```python
from build123d import *

# Parameters (mm, degrees)
F0_W     = 50
F0_H     = 25
F1_DEPTH = 10
F2_R     = 4
F3_W     = 5
F3_H     = 15
F4_DEPTH = 25
F5_R     = 1
F6_R     = 3.6231488333
F6_R_2   = 2.5645914907
F7_DEPTH = 1.5


with BuildPart() as f1:
    # F0 (on Top) → F1 (new body)
    with BuildSketch(Plane.XY):
        Rectangle(F0_W, F0_H)
    extrude(amount=F1_DEPTH)

    # F2
    f2_edges = [f1.edges().sort_by_distance(p)[0] for p in [
        (-25, -12.5, 5),
        (25, -12.5, 5),
        (25, 12.5, 5),
        (-25, 12.5, 5),
    ]]
    fillet(f2_edges, radius=F2_R)

    # F3 (on face) → F4 (cut)
    with BuildSketch(Plane.XY.offset(10)):
        with Locations((-18.5, 0)):
            Rectangle(F3_W, F3_H)
    extrude(amount=-F4_DEPTH, mode=Mode.SUBTRACT)

    # F5
    f5_edges = [f1.edges().sort_by_distance(p)[0] for p in [
        (-21, 7.5, 5),
        (-21, -7.5, 5),
        (-16, 7.5, 5),
        (-16, -7.5, 5),
    ]]
    fillet(f5_edges, radius=F5_R)

    # F6 (on face) → F7 (join)
    with BuildSketch(Plane.XY.offset(10)):
        with BuildLine():
            ThreePointArc((0, -8.4754349664), (4.4343331639, -0.0092051923), (0, 8.4570245817))
            ThreePointArc((0, 8.4570245817), (-4.7324505421, -0.0092051923), (0, -8.4754349664))
        make_face()
        with BuildLine():
            ThreePointArc((0, -7.3103578761), (-3.8122546037, 0.107302476), (0, 7.524962828))
            ThreePointArc((0, 7.524962828), (3.6492929607, 0.107302476), (0, -7.3103578761))
        make_face(mode=Mode.SUBTRACT)
        Circle(F6_R)
        Circle(F6_R_2, mode=Mode.SUBTRACT)
        with BuildLine():
            Line((-7.5879783359, -7.5879783359), (-3.4245205097, -6.8479519513))
            ThreePointArc((-3.4245205097, -6.8479519513), (-5.2850781661, -5.385812279), (-6.795665493, -3.5643696799))
            Line((-6.795665493, -3.5643696799), (-7.5879783359, -7.5879783359))
        make_face()
        with BuildLine():
            ThreePointArc((-7.2637349367, -2.4207315873), (-7.545458995, -0.0712297744), (-7.3256511241, 2.2848711815))
            Line((-7.3256511241, 2.2848711815), (-10.7310218737, 0))
            Line((-10.7310218737, 0), (-7.2637349367, -2.4207315873))
        make_face()
        with BuildLine():
            Line((-3.5643696799, 6.795665493), (-7.5879783359, 7.5879783359))
            Line((-7.5879783359, 7.5879783359), (-6.8479519513, 3.4245205097))
            ThreePointArc((-6.8479519513, 3.4245205097), (-5.385812279, 5.2850781661), (-3.5643696799, 6.795665493))
        make_face()
    extrude(amount=F7_DEPTH)


solid = f1.part
```
Could you check a few things on this model? Use its own coordinates, in mm. A direction names the side the tool comes from. Round coordinates to 2 decimals unless told otherwise and drop trailing zeros. Write each loop counter-clockwise with the first axis right and the second up, starting at its lowest first coordinate (ties: lowest second). Pieces come first, ordered by that corner, then holes.
(1) Thinking about a two-plate mould opening in X: for faces 1 (the face through (-19, 7.5, 5)), 2 (the face through (-23.859, 11.297, 5.07)), 3 (the face through (0, 0, 0)), which applies, +X half, -X half, draft (parallel to the pull), parting line (faces both ways), or undercut?
Findings below:
face 1: undercut
face 2: -X half
face 3: draft
(2) Suppose I cut it at A-A on y = 4.75. Write out the boundary of the cut face in (x, z).
Findings below:
outline: (-25, 0) - (-21, 0) - (-21, 10) - (-25, 10) - close; (-16, 0) - (25, 0) - (25, 10) - (3.27, 10) - (3.27, 11.5) - (2.42, 11.5) - (2.42, 10) - (-2.54, 10) - (-2.54, 11.5) - (-3.52, 11.5) - (-3.52, 10) - (-5.87, 10) - (-5.87, 11.5) - (-7.08, 11.5) - (-7.08, 10) - (-16, 10) - close
(3) Suppose I cut it at B-B on z = 4.5. Write out the boundary of the cut face in (x, y), and give its area (3 significant figures).
Findings below:
outline: (-25, -8.5) arc R4 ccw to (-21, -12.5) - (21, -12.5) arc R4 ccw to (25, -8.5) - (25, 8.5) arc R4 ccw to (21, 12.5) - (-21, 12.5) arc R4 ccw to (-25, 8.5) - close; hole (-21, -6.5) arc R1 ccw to (-20, -7.5) - (-17, -7.5) arc R1 ccw to (-16, -6.5) - (-16, 6.5) arc R1 ccw to (-17, 7.5) - (-20, 7.5) arc R1 ccw to (-21, 6.5) - close
area: 1,160 mm2
(4) Suppose I cut it at D-D on x = 17. Write out the boundary of the cut face in (y, z).
Findings below:
outline: (-12.5, 0) - (12.5, 0) - (12.5, 10) - (-12.5, 10) - close
(5) For pin 1 (8 mm diameter, centred on x = 0.5, y = -6, fed in from +Z); pin 2 (7.5 mm diameter, centred on x = 11, y = 1, fed in from +Z), each with a flat end and sliding along its axis, tell me the tip position at first contact or that it passes through.
Findings below:
pin 1: stops at z = 11.5
pin 2: stops at z = 10
(6) If I drill on probe 1 along X at (y, z) = (6.25, 4.75); probe 2 along Z at (x, y) = (-2, 11.75); probe 3 along X at (y, z) = (11.5, 6.5), over which ranges is the centre line in solid material (lowest first)?
Findings below:
probe 1: x = -25 to -21, -16 to 25
probe 2: z = 0 to 10
probe 3: x = -23.65 to 23.65
(7) Suppose I cut it at C-C on x = -8.5. Write out the boundary of the cut face in (y, z), and give its area (3 significant figures).
Findings below:
outline: (-12.5, 0) - (12.5, 0) - (12.5, 10) - (1.5, 10) - (1.5, 11.5) - (-1.56, 11.5) - (-1.56, 10) - (-12.5, 10) - close
area: 255 mm2
(8) Which directions (+Z, -Z, +X, -X, +Y, -Y) give clear straight access to the entire face, cutting with the end or side of a thin tool? Please do faces 4 (the face through (-6, -6, 11.5)), 5 (the face through (-16, 0, 5)), 6 (the face through (-3, 3, 10)).
Findings below:
face 4: +Z, +X, -X, +Y, -Y
face 5: +Z, -Z
face 6: +Z
